Part model, mm, in its own coordinate system. Face numbers are marked on the shaded views. A direction names the side the tool comes from. Coordinates: 2 decimals unless noted, no trailing zeros. Order: outer loops, then holes, each group sorted by start corner. A loop starts at its lowest first (then second) coordinate and runs counter-clockwise, first axis right, second up.
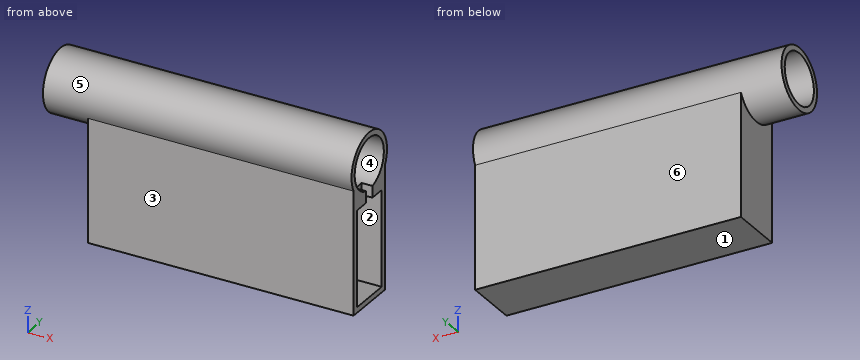
```python
from build123d import *

# Parameters (mm, degrees)
F0_R     = 17.78
F0_R_2   = 14.605
F1_DEPTH = 177.8
F2_W     = 25
F2_H     = 55
F3_DEPTH = 150
F5_DEPTH = 3.175
F6_W     = 6.35
F6_H     = 13.6751307396
F7_DEPTH = 6.35


with BuildPart() as f1:
    # F0 (on Right) → F1 (new body)
    with BuildSketch(Plane.YZ):
        Circle(F0_R)
        Circle(F0_R_2, mode=Mode.SUBTRACT)
    extrude(amount=-F1_DEPTH)

    # F2 (on Right) → F3 (join)
    with BuildSketch(Plane.YZ):
        Polygon((-7.21e-08, -17.78), (-15.675, -17.78), (-15.675, -79.13), (15.675, -79.13), (15.675, -17.78), align=None)
        with Locations((0, -48.455)):
            Rectangle(F2_W, F2_H, mode=Mode.SUBTRACT)
        with BuildLine():
            Line((-15.675, -8.39182787), (-15.675, -17.78))
            Line((-15.675, -17.78), (-7.21e-08, -17.78))
            ThreePointArc((-7.21e-08, -17.78), (-9.1356910412, -15.2534438472), (-15.675, -8.39182787))
        make_face()
        with BuildLine():
            ThreePointArc((15.675, -8.39182787), (9.1356909794, -15.2534438842), (-7.21e-08, -17.78))
            Line((-7.21e-08, -17.78), (15.675, -17.78))
            Line((15.675, -17.78), (15.675, -8.39182787))
        make_face()
    extrude(amount=-F3_DEPTH)

    # F4 (on face) → F5 (join)
    with BuildSketch(Plane(origin=(-150, 0, 0), x_dir=(0, -1, 0), z_dir=(-1, 0, 0))):
        Polygon((-15.675, -17.78), (-15.675, -79.13), (15.675, -79.13), (15.675, -17.78), (0, -17.78), align=None)
        with BuildLine():
            Line((-15.675, -8.39182787), (-15.675, -17.78))
            Line((-15.675, -17.78), (0, -17.78))
            ThreePointArc((0, -17.78), (-9.1356910103, -15.2534438657), (-15.675, -8.39182787))
        make_face()
        with BuildLine():
            Line((0, -17.78), (15.675, -17.78))
            Line((15.675, -17.78), (15.675, -8.39182787))
            ThreePointArc((15.675, -8.39182787), (9.1356910103, -15.2534438657), (0, -17.78))
        make_face()
    extrude(amount=F5_DEPTH)

    # F6 (on Right) → F7 (cut)
    with BuildSketch(Plane.YZ):
        with Locations((0, -18.0660898343)):
            Rectangle(F6_W, F6_H)
    extrude(amount=-F7_DEPTH, mode=Mode.SUBTRACT)


solid = f1.part
```
(1) Slice it at C-C, the plane x = -123.5. Give the cut face in (y, z) (3 decimals), then the cut area to 3 significant figures.
(2) Drop flat-ended pins along their axis: pin 1 (3 mm diameter, centred on y = -1.5, z = -18, fed in from +X); pin 2 (12 mm diameter, centred on y = 3, z = -24, fed in from +X); pin 3 (4 mm diameter, centred on y = -3, z = -56, fed in from +X); pin 4 (4 mm diameter, centred on x = -37, y = 11.5, fed in from +Z). Give the stop position or say it passes through.
(3) Probe line 1 (Z direction, x = -52, y = 0) (3 decimals); line 2 (Y direction, x = -59.5, z = 0) (3 decimals); line 3 (Y direction, x = -6.5, z = -52) (3 decimals). List the from-to ranges inside material, lowest first.
(4) Pull direction Z, two halves, no side cores. Call the marked faces 4, 5 and 6: +Z half, -Z half, draft (parallel to the pull), parting line (faces both ways), or undercut.
(5) Slice it at A-A, the plane z = 0. Give the cut face in (x, y) (3 decimals), then the cut area to 3 significant figures.
(6) Slice it at D-D, the plane z = -23.5. Give the cut face in (x, y) (3 decimals).
(7) Tool access for the marked faces 1, 2 and 3: list every direction of +Z, -Z, +X, -X, +Y, -Y with a clear straight run to the whole face (end or side of a thin tool).
(8) Slice it at B-B, the plane y = 0. Give the cut face in (x, z) (3 decimals), then the cut area to 3 significant figures.
Here are the results:
1. outline: (-15.675, -79.13) - (15.675, -79.13) - (15.675, -8.392) arc R17.78 ccw (long way) to (-15.675, -8.392) - close; hole circle Ø29.21 at (0, 0); hole (-12.5, -75.955) - (12.5, -75.955) - (12.5, -20.955) - (-12.5, -20.955) - close
1. area: 956 mm2
2. pin 1: stops at x = -6.35
2. pin 2: stops at x = 0
2. pin 3: stops at x = -150
2. pin 4: stops at z = 15.03
3. line 1: z = -79.13 to -75.955, -20.955 to -14.605, 14.605 to 17.78
3. line 2: y = -17.78 to -14.605, 14.605 to 17.78
3. line 3: y = -15.675 to -12.5, 12.5 to 15.675
4. face 4: undercut
4. face 5: parting line
4. face 6: draft
5. outline: (-177.8, -17.78) - (0, -17.78) - (0, -14.605) - (-177.8, -14.605) - close; (-177.8, 14.605) - (0, 14.605) - (0, 17.78) - (-177.8, 17.78) - close
5. area: 1,130 mm2
6. outline: (-153.175, -15.675) - (0, -15.675) - (0, -12.5) - (-150, -12.5) - (-150, 12.5) - (0, 12.5) - (0, 15.675) - (-153.175, 15.675) - close
7. face 1: -Z, +X, -X, +Y, -Y
7. face 2: +X
7. face 3: -Z, +X, -X, -Y
8. outline: (-177.8, -17.78) - (-153.175, -17.78) - (-153.175, -79.13) - (0, -79.13) - (0, -75.955) - (-150, -75.955) - (-150, -20.955) - (-6.35, -20.955) - (-6.35, -14.605) - (-177.8, -14.605) - close; (-177.8, 14.605) - (0, 14.605) - (0, 17.78) - (-177.8, 17.78) - close
8. area: 2,240 mm2
